Can you work these out from the model? Positions are in its coordinate system, mm. Face numbers are marked on the shaded views. A direction names the side the tool comes from. Coordinates: 2 decimals unless noted, no trailing zeros. Order: outer loops, then holes, each group sorted by start corner. A loop starts at its lowest first (then second) coordinate and runs counter-clockwise, first axis right, second up. Notation, with made-up numbers: M 43.25,13 L 68.25,13 A25 ccw 68.25,37 Z; hole C 13,-32 d9. An arc over 180 degrees is marked long. Answer as a JSON object with one key per item and string values.
from build123d import *

# Parameters (mm, degrees)
F0_W     = 7.8990748152
F0_H     = 28.538595885
F0_W_2   = 6.6250311211
F0_H_2   = 28.0289780349
F1_DEPTH = 12.7
F2_R     = 5.08


# Not quite as in the source:
# - two fillets or chamfers of one size are made in one step


with BuildPart() as f1:
    # F0 (on Front) → F1 (new body)
    with BuildSketch(Plane.XZ):
        Polygon((10.9567856416, 73.384962976), (0, 73.384962976), (0, 28.538595885), (0, 0), (0, -76.9523009658), (10.9567856416, -76.9523009658), (10.9567856416, -63.2497891784), (10.9567856416, -57.5868189335), (10.9567856416, 0), (10.9567856416, 28.0289780349), align=None)
        with Locations((-3.9495374076, 14.2692979425)):
            Rectangle(F0_W, F0_H)
        with Locations((14.2693012021, 14.0144890174)):
            Rectangle(F0_W_2, F0_H_2)
        Polygon((-7.8990748152, 0), (-7.8990748152, 28.538595885), (-21.1491379887, -25.4808943719), (-25.4754136512, -24.4197324549), (-25.7356986403, -29.0482211858), (-11.9106527418, -29.0482211858), (-7.8990748152, -29.0482211858), align=None)
        Polygon((10.9567856416, -63.2497891784), (10.9567856416, -76.9523009658), (65.48589468, -76.9523009658), (59.3128465116, -63.2497891784), align=None)
        Polygon((-25.7356986403, -29.0482211858), (-25.4754136512, -24.4197324549), (-25.4754136512, -11.2115936354), (-35.4184396565, -11.2115936354), (-35.4184396565, -25.9905140847), (-40.5146181583, -25.9905140847), (-53.649477917, -35.9711753499), (-46.4077852666, -36.2483747303), (-46.4077852666, -34.144397825), (-40.0049984455, -34.144397825), (-35.4184396565, -34.3199633062), (-35.4184396565, -37.3197160661), (-25.7356986403, -37.3197160661), (-25.7356986403, -34.7485020757), (-11.9106527418, -34.7485020757), (-11.9106527418, -29.0482211858), align=None)
    extrude(amount=F1_DEPTH)

    # F2
    f2_edges = [f1.edges().sort_by_distance(p)[0] for p in [
        (-35.41844, -12.7, -18.601054),
        (10.956786, -12.7, -31.624895),
        (0, -12.7, 50.961779),
        (0, -12.7, -38.47615),
        (0, 0, 50.961779),
        (-14.524106, -12.7, 1.528851),
        (-7.899075, 0, -14.524111),
        (62.399371, -12.7, -70.101045),
        (10.956786, 0, 50.706971),
        (10.956786, -12.7, 50.706971),
    ]]
    fillet(f2_edges, radius=F2_R)


solid = f1.part
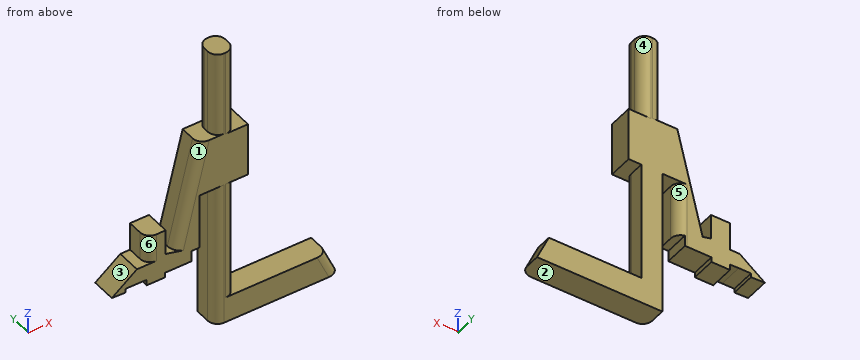
Item 1: Which directions (+Z, -Z, +X, -X, +Y, -Y) give clear straight access to the entire face, cutting with the end or side of a thin tool? Please do the marked faces 4, 5 and 6.
Answers follow:
{"face 4": "+Z, +X, +Y", "face 5": "-Z, +Y", "face 6": "+Z, -X, -Y"}
Item 2: I want a section at A-A, the plane x = 16. Write out the boundary of the cut face in (y, z), plus the area to 3 significant figures.
Answers follow:
{"outline": "M -12.7,-76.95 L 0,-76.95 L 0,-63.25 L -12.7,-63.25 Z; M -12.7,0 L 0,0 L 0,28.03 L -12.7,28.03 Z", "area": "530 mm^2"}
Item 3: Please list where these lines run through material, in increasing order: line 1 (Z direction, x = 13.5, y = -2); line 2 (X direction, y = -7, z = -13); line 3 (X direction, y = -6, z = -14.5).
Answers follow:
{"line 1": "z = -76.95 to -63.25, 0 to 28.03", "line 2": "x = -35.42 to -25.48, -18.09 to -7.9, 0 to 10.96", "line 3": "x = -35.42 to -25.48, -18.46 to -7.9, 0 to 10.96"}
Item 4: If we mould it in two halves opening along X, with no side actions, what happens to the marked faces 1, 2 and 3? For each: pulls with the +X half, pulls with the -X half, needs draft (parallel to the pull), parting line crosses it, or undercut.
Answers follow:
{"face 1": "undercut", "face 2": "needs draft", "face 3": "pulls with the -X half"}
Item 5: I'm going to push flat-ended pins straight in: pin 1 (6.5 mm diameter, centred on y = -5.5, z = -15.5, fed in from +X); pin 2 (1.7 mm diameter, centred on y = -9, z = -35.5, fed in from +X); pin 3 (4 mm diameter, centred on x = 1.5, z = 49, fed in from +Y). Where does each tip first touch, or does it pass through?
Answers follow:
{"pin 1": "stops at x = 10.96", "pin 2": "stops at x = 10.93", "pin 3": "stops at y = -0.25"}
Item 6: I want a section at B-B, the plane z = 63. Write out the boundary of the cut face in (x, y).
Answers follow:
{"outline": "M 0,-7.62 A5.08 ccw 5.08,-12.7 L 5.88,-12.7 A5.08 ccw 10.96,-7.62 L 10.96,-5.08 A5.08 ccw 5.88,0 L 5.08,0 A5.08 ccw 0,-5.08 Z"}
